Build history of the part. All positions in model axes, mm. A direction names the side the tool comes from. Coordinates: 2 decimals unless noted, no trailing zeros. Loops run counter-clockwise (first coordinate to the right, second up) from the corner with the lowest first, then second, coordinate; pieces in that order, holes last.
Item 1: Cut at B-B (z = -5.5). List the corners of the cut face in (x, y).
Item 2: 3-axis set-ups, long thin cutter, end or side, ignore diameter. For faces 1 (the face through (-0.2, 11.5, 11.7)), 2 (the face through (6, 10, -3.491)): which of +Z, -Z, +X, -X, +Y, -Y reach the whole face in a straight line?
Item 3: Cut at A-A (x = 0). List the corners of the cut face in (y, z), and give its area (3 significant figures).
Item 4: Mould opens along X. For faces 3 (the face through (3.997, 10, -6)), 4 (the face through (-0.137, 11.493, -9.214)), 5 (the face through (6, 10, -8.491)), 6 (the face through (7.889, 10, -6)) say: released by +X, released by -X, zero draft, split by the parting line, or undercut.
Item 5: Cut at D-D (y = 11.4). List the corners of the cut face in (x, z), and give its area (3 significant figures).
Item 6: Cut at C-C (x = 5). List the corners of the cut face in (y, z).
Item 7: Flat gauge pins, fed straight in: pin 1 (2 mm diameter, centred on y = 9.5, z = -5, fed in from +X); pin 2 (5 mm diameter, centred on x = 0.5, z = -7.5, fed in from -Y). Where does each tip first touch, or does it go through?
Item 8: Drill centre lines: line 1 along Z through (x, y) = (0, 11.5); line 2 along Y through (x, z) = (5.75, -10); line 3 along X through (y, z) = (11.1, -9.75). Where is each one in solid material? Low to high.
from build123d import *

# Parameters (mm, degrees)
SKETCH_2_R          = 12
SKETCH_1_R          = 12.5
CUT_EXTRUDE_1_DEPTH = 12.0000001
SKETCH_5_W          = 13
SKETCH_5_H          = 6
CUT_EXTRUDE_2_DEPTH = 5
SKETCH_6_W          = 2.476692414
SKETCH_6_H          = 6.83521307
CUT_EXTRUDE_3_DEPTH = 20
CUT_EXTRUDE_4_DEPTH = 5
SKETCH_9_R          = 0.630926361
EXTRUDE_1_DEPTH     = 1
SKETCH_11_W         = 27.446294714
SKETCH_11_H         = 11.793449851
CUT_EXTRUDE_5_DEPTH = 21.75
SKETCH_10_W         = 3.891529141
SKETCH_10_H         = 5
EXTRUDE_2_DEPTH     = 2.5


with BuildPart() as part:
    # 草图2 → 放样1 section 0
    with BuildSketch(Plane(origin=(0, 11, 0), x_dir=(1, 0, 0), z_dir=(0, 1, 0))):
        Circle(SKETCH_2_R)
    # 草图1 → 放样1 section 1
    with BuildSketch(Plane(origin=(0, 0, 0), x_dir=(1, 0, 0), z_dir=(0, 1, 0))):
        Circle(SKETCH_1_R)
    loft()

    # 草图4 → 切除-拉伸1 (cut, through all)
    with BuildSketch(Plane(origin=(0, 0, 0), x_dir=(1, 0, 0), z_dir=(0, 1, 0))):
        with BuildLine():
            Line((-1.352272566, -2.5), (-1.352272566, -2.102702762))
            ThreePointArc((-1.352272566, -2.102702762), (0.025010963, 2.499874887), (1.309931483, -2.12933781))
            Line((1.309931483, -2.12933781), (1.309931483, -2.5))
            Line((1.309931483, -2.5), (8, -2.5))
            Line((8, -2.5), (8, -7.5))
            Line((8, -7.5), (-8, -7.5))
            Line((-8, -7.5), (-8, -2.5))
            Line((-8, -2.5), (-1.352272566, -2.5))
        make_face()
    extrude(amount=CUT_EXTRUDE_1_DEPTH, mode=Mode.SUBTRACT)

    # 草图5 → 切除-拉伸2 (cut)
    with BuildSketch(Plane(origin=(0, 11, 0), x_dir=(1, 0, 0), z_dir=(0, 1, 0))):
        with Locations((0, 5.991032562)):
            Rectangle(SKETCH_5_W, SKETCH_5_H)
        with BuildLine():
            Line((7.947410488, 8.991032562), (6.5, 8.991032562))
            Line((6.5, 8.991032562), (6.5, 2.991032562))
            Line((6.5, 2.991032562), (11.621261731, 2.991032562))
            ThreePointArc((11.621261731, 2.991032562), (10.233925596, 6.266320045), (7.947410488, 8.991032562))
        make_face()
        with BuildLine():
            Line((15.348611284, 8.991032562), (7.947410488, 8.991032562))
            ThreePointArc((7.947410488, 8.991032562), (10.233925596, 6.266320045), (11.621261731, 2.991032562))
            Line((11.621261731, 2.991032562), (15.348611284, 2.991032562))
            Line((15.348611284, 2.991032562), (15.348611284, 8.991032562))
        make_face()
    extrude(amount=-CUT_EXTRUDE_2_DEPTH, mode=Mode.SUBTRACT)

    # 草图6 → 切除-拉伸3 (cut, symmetric)
    with BuildSketch(Plane(origin=(0, 0, 0), x_dir=(0, 0, -1), z_dir=(1, 0, 0))):
        with Locations((0, 8.790545757)):
            Rectangle(SKETCH_6_W, SKETCH_6_H)
    extrude(amount=CUT_EXTRUDE_3_DEPTH, both=True, mode=Mode.SUBTRACT)

    # 草图7 → 切除-拉伸4 (cut)
    with BuildSketch(Plane(origin=(0, 11, 0), x_dir=(1, 0, 0), z_dir=(0, 1, 0))):
        Polygon((-5.998196858, 2.991032562), (-5.998196858, -3.96939498), (-8, -3.96939498), (-9.46939498, -2.5), (-9.46939498, 3.910589128), (-7.645587141, 5.734396966), (-6.5, 5.734396966), align=None)
    extrude(amount=-CUT_EXTRUDE_4_DEPTH, mode=Mode.SUBTRACT)

    # 草图9 → 凸台-拉伸1 (add)
    with BuildSketch(Plane(origin=(0, 11, 0), x_dir=(1, 0, 0), z_dir=(0, 1, 0))):
        with BuildLine():
            Line((-10, 6.073713856), (-10, -6.073713856))
            ThreePointArc((-10, -6.073713856), (0, -11.7), (10, -6.073713856))
            Line((10, -6.073713856), (10, 6.073713856))
            ThreePointArc((10, 6.073713856), (0, 11.7), (-10, 6.073713856))
        make_face()
        with Locations((0, 9.829977892)):
            Circle(SKETCH_9_R, mode=Mode.SUBTRACT)
    extrude(amount=EXTRUDE_1_DEPTH)

    # 草图11 → 切除-拉伸5 (cut, symmetric)
    with BuildSketch(Plane(origin=(0, 0, 0), x_dir=(0, 0, -1), z_dir=(1, 0, 0))):
        with Locations((-0.090881771, 5.103275074)):
            Rectangle(SKETCH_11_W, SKETCH_11_H)
    extrude(amount=CUT_EXTRUDE_5_DEPTH, both=True, mode=Mode.SUBTRACT)

    # 草图10 → 凸台-拉伸2 (add)
    with BuildSketch(Plane.XZ.offset(-11)):
        with Locations((5.943222156, -5.991032562)):
            Rectangle(SKETCH_10_W, SKETCH_10_H)
    extrude(amount=EXTRUDE_2_DEPTH)


solid = part.part
Filled sheet:
1. outline: (-10, 11) - (4, 11) - (4, 8.5) - (7.89, 8.5) - (7.89, 11) - (10, 11) - (10, 12) - (-10, 12) - close
2. face 1: +Z, +Y, -Y
2. face 2: +Z, +X, -X, -Y
3. outline: (11, -11.7) - (12, -11.7) - (12, -10.46) - (11, -10.46) - close; (11, -9.2) - (12, -9.2) - (12, 11.7) - (11, 11.7) - close
3. area: 22.1 mm2
4. face 3: released by -X
4. face 4: undercut
4. face 5: zero draft
4. face 6: released by +X
5. outline: (-10, -6.07) arc R11.7 ccw to (10, -6.07) - (10, 6.07) arc R11.7 ccw to (-10, 6.07) - close; hole circle Ø1.26 at (0, -9.83)
5. area: 401 mm2
6. outline: (8.5, -8.49) - (11, -8.49) - (11, -10.58) - (12, -10.58) - (12, 10.58) - (11, 10.58) - (11, -3.49) - (8.5, -3.49) - close
7. pin 1: stops at x = 7.89
7. pin 2: stops at y = 11
8. line 1: z = -11.7 to -10.46, -9.2 to 11.7
8. line 2: y = 11 to 12
8. line 3: x = -6.47 to -0.63, 0.63 to 6.47
